from build123d import *

# Parameters (mm, degrees)
CYLINDER001_R          = 1.98
CYLINDER001_DEPTH      = 11
CYLINDER001_ROLL_ANGLE = -90
CYLINDER004_R          = 3.5
CYLINDER004_DEPTH      = 3
CYLINDER004_ROLL_ANGLE = 90
CYLINDER_R             = 5.5
CYLINDER_DEPTH         = 8
CYLINDER_ROLL_ANGLE    = -90


with BuildPart() as f_10_32_tap_hole:
    # Cylinder001 → Cylinder001 (new body)
    with BuildSketch(Plane.XY):
        Circle(CYLINDER001_R)
    extrude(amount=CYLINDER001_DEPTH)


with BuildPart() as f_10_32_tap_hole_1:
    # Cylinder001 roll: moved
    add(f_10_32_tap_hole.part.rotate(Axis((0, 0, 0), (1, 0, 0)), CYLINDER001_ROLL_ANGLE))


with BuildPart() as f_10_32_tap_hole_2:
    # Cylinder001 placement: moved
    add(f_10_32_tap_hole_1.part.moved(Location((17.5, -3, 6))))


with BuildPart() as thin_neck:
    # Cylinder004 → Cylinder004 (new body)
    with BuildSketch(Plane.XY):
        Circle(CYLINDER004_R)
    extrude(amount=CYLINDER004_DEPTH)


with BuildPart() as thin_neck_1:
    # Cylinder004 roll: moved
    add(thin_neck.part.rotate(Axis((0, 0, 0), (1, 0, 0)), CYLINDER004_ROLL_ANGLE))


with BuildPart() as thin_neck_2:
    # Cylinder004 placement: moved
    add(thin_neck_1.part.moved(Location((17.5, 0, 6))))


with BuildPart() as f_10_32_support_neck_and_taphole:
    # Cylinder → Cylinder (new body)
    with BuildSketch(Plane.XY):
        Circle(CYLINDER_R)
    extrude(amount=CYLINDER_DEPTH)


with BuildPart() as f_10_32_support_neck_and_taphole_1:
    # Cylinder roll: moved
    add(f_10_32_support_neck_and_taphole.part.rotate(Axis((0, 0, 0), (1, 0, 0)), CYLINDER_ROLL_ANGLE))


with BuildPart() as f_10_32_support_neck_and_taphole_2:
    # Cylinder placement: moved
    add(f_10_32_support_neck_and_taphole_1.part.moved(Location((17.5, 0, 6))))

    # Fusion002: union thin_neck
    add(thin_neck_2.part)

    # Cut: cut 10-32_tap_hole
    add(f_10_32_tap_hole_2.part, mode=Mode.SUBTRACT)


solid = f_10_32_support_neck_and_taphole_2.part
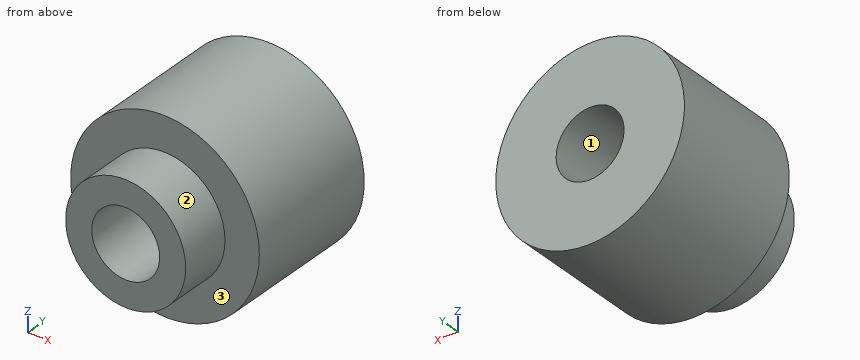
Design review of the part built by this model. Coordinates are the model's own, in mm. Face numbers are marked on the shaded views. Round coordinates to 2 decimals unless told otherwise and drop trailing zeros. Write each loop counter-clockwise with the first axis right and the second up, starting at its lowest first coordinate (ties: lowest second). Pieces come first, ordered by that corner, then holes. Notation, with made-up numbers: (76, 26) -> (83, 26) arc R29 cw to (83, 62) -> close; hole circle Ø7 at (-35, 35). An arc over 180 degrees is marked (long way). One line per item, written item: value. Start each with the question number.
Q1. Add section A-A (z = 6). Give the boundary of the cut face in (x, y).
Q2. Add section D-D (x = 19.75). Give the boundary of the cut face in (y, z).
Q3. To check wall thickness, follow probe 1 along Z at (x, y) = (17.5, 2.75); probe 2 along X at (y, z) = (2.5, 6); probe 3 along Y at (x, z) = (15, 9). State the ranges of each line that lie inside material, in increasing order.
Q4. Add section B-B (x = 17.5). Give the boundary of the cut face in (y, z), then the cut area to 3 significant figures.
Q5. The part is to be moulded in two halves that separate along Z. For the marked faces 1, 2 and 3, say which applies: pulls with the +Z half, pulls with the -Z half, needs draft (parallel to the pull), parting line crosses it, or undercut.
Q6. Insertion check: P1, Ø4, axis at x = 21.5, y = 5, coming from the -Z side. The pin has a flat end and moves straight along its axis. Give the tip position at first contact, or say it passes through.
Q7. Add section C-C (y = 3.75). Give the boundary of the cut face in (x, z).
Response:
1. outline: (12, 0) -> (14, 0) -> (14, -3) -> (15.52, -3) -> (15.52, 8) -> (12, 8) -> close; (19.48, -3) -> (21, -3) -> (21, 0) -> (23, 0) -> (23, 8) -> (19.48, 8) -> close
2. outline: (-3, 3.32) -> (0, 3.32) -> (0, 0.98) -> (8, 0.98) -> (8, 11.02) -> (0, 11.02) -> (0, 8.68) -> (-3, 8.68) -> close
3. probe 1: z = 0.5 to 4.02, 7.98 to 11.5
3. probe 2: x = 12 to 15.52, 19.48 to 23
3. probe 3: y = 0 to 8
4. outline: (-3, 2.5) -> (0, 2.5) -> (0, 0.5) -> (8, 0.5) -> (8, 4.02) -> (-3, 4.02) -> close; (-3, 7.98) -> (8, 7.98) -> (8, 11.5) -> (0, 11.5) -> (0, 9.5) -> (-3, 9.5) -> close
4. area: 65.4 mm^2
5. face 1: undercut
5. face 2: parting line crosses it
5. face 3: needs draft
6. P1: stops at z = 0.88
7. outline: circle Ø11 at (17.5, 6); hole circle Ø3.96 at (17.5, 6)
